from build123d import *

# Parameters (mm, degrees)
SKETCH1_R           = 3.175
BOSS_EXTRUDE1_DEPTH = 3.048


with BuildPart() as part:
    # Sketch1 → Boss-Extrude1 (new, symmetric)
    with BuildSketch(Plane(origin=(0, 0, 0), x_dir=(1, 0, 0), z_dir=(0, 1, 0))):
        with BuildLine():
            Line((34.700549349, -12.916534941), (61.399556839, -22.854667611))
            ThreePointArc((61.399556839, -22.854667611), (55.420174256, -34.940602415), (47.093148029, -45.546424892))
            ThreePointArc((47.093148029, -45.546424892), (15.086508303, -14.560725649), (-28.536322062, -23.593289791))
            Line((-28.536322062, -23.593289791), (-50.492501165, -41.746242199))
            ThreePointArc((-50.492501165, -41.746242199), (-57.969536443, -30.52497758), (-62.990935022, -18.010650091))
            ThreePointArc((-62.990935022, -18.010650091), (-20.153212462, -5.78493662), (-6.164227287, 36.509824732))
            Line((-6.164227287, 36.509824732), (-10.907055674, 64.600909809))
            ThreePointArc((-10.907055674, 64.600909809), (2.549362187, 65.465579995), (15.897786993, 63.557074983))
            ThreePointArc((15.897786993, 63.557074983), (5.066704158, 20.34566227), (34.700549349, -12.916534941))
        make_face()
        Circle(SKETCH1_R, mode=Mode.SUBTRACT)
    extrude(amount=BOSS_EXTRUDE1_DEPTH, both=True)


solid = part.part
Work out the finished part from the listing and answer in its coordinate system (mm). Round coordinates to 2 decimals unless told otherwise and drop trailing zeros. Write each loop counter-clockwise with the first axis right and the second up, starting at its lowest first coordinate (ties: lowest second). Pieces come first, ordered by that corner, then holes.
1) A cutting plane is placed at D-D (x = 40.5). Give the vertices of the cut face in (y, z), plus the area to 3 significant figures.
2) A cutting plane is placed at B-B (z = 0). Give the vertices of the cut face in (x, y) (3 decimals), plus the area to 3 significant figures.
3) The mould has two halves that part along X. Classify faces 1 (the flat face through (47.863, 0.043, 17.816)), 2 (the flat face through (-8.502, 0.043, -50.359)), 3 (the flat face through (-39.36, 0.04, 32.54)): pulls with the +X half, pulls with the -X half, needs draft (parallel to the pull), parting line crosses it, or undercut.
4) Given pin 1 Ø10 at (x, z) = (0, 0) entering from +Y; pin 2 Ø2 at (y, z) = (-1, 10.5) entering from +X; pin 3 Ø3 at (y, z) = (-1, -35) entering from -X; pin 4 Ø3 at (x, y) = (-15.5, -1) entering from +Z, each flat-ended and moving along its own axis, determine where each tip first touches the part or whether it passes through.
5) A cutting plane is placed at C-C (x = 0). Give the vertices of the cut face in (y, z) (3 decimals).
6) Straight lines are drawn through the part: line 1 (X direction, y = -0.75, z = 0) (3 decimals); line 2 (Z direction, x = 8, y = 0.5); line 3 (Z direction, x = 0, y = 1.75) (3 decimals). For each, find the intervals that lie inside material, in ascending order.
Completed:
1. outline: (-3.05, 15.08) - (3.05, 15.08) - (3.05, 32.53) - (-3.05, 32.53) - close
1. area: 106 mm2
2. outline: (-15.029, -3.048) - (-3.175, -3.048) - (-3.175, 3.048) - (-15.029, 3.048) - close; (3.175, -3.048) - (15.787, -3.048) - (15.787, 3.048) - (3.175, 3.048) - close
2. area: 149 mm2
3. face 1: pulls with the +X half
3. face 2: pulls with the -X half
3. face 3: undercut
4. pin 1: stops at y = 3.05
4. pin 2: stops at x = 31.3
4. pin 3: stops at x = -6.16
4. pin 4: stops at z = 16.54
5. outline: (-3.048, -65.515) - (3.048, -65.515) - (3.048, -3.175) - (-3.048, -3.175) - close; (-3.048, 3.175) - (3.048, 3.175) - (3.048, 12.707) - (-3.048, 12.707) - close
6. line 1: x = -15.029 to -3.175, 3.175 to 15.787
6. line 2: z = -65.02 to -51.52, -11.92 to 13.08
6. line 3: z = -65.515 to -3.175, 3.175 to 12.707
